Source: CAD feature listing. Evaluate the final solid. Frame: model axes, mm. A direction names the side the tool comes from. Give positions to 0.01 mm unless a question says otherwise; leave off trailing zeros. Order: outer loops, then holes, each group sorted by start corner. A loop starts at its lowest first (then second) coordinate and runs counter-clockwise, first axis right, second up. Notation, with made-up numbers: (78.25, -26) -> (115.25, -26) arc R8 cw to (115.25, -21) -> close; hole circle Ø10 at (-4.5, 45.25). An arc over 180 degrees is marked (long way). Answer in a Markdown table with one row per item.
```python
from build123d import *

# Parameters (mm, degrees)
SKETCH1_R           = 20
BOSS_EXTRUDE1_DEPTH = 2
SKETCH2_R           = 18.25
BOSS_EXTRUDE2_DEPTH = 10
BOSS_EXTRUDE2_TAPER = 3
SKETCH3_R           = 11.5
BOSS_EXTRUDE3_DEPTH = 9.5
FILLET1_R           = 1


with BuildPart() as part:
    # Sketch1 → Boss-Extrude1 (new body)
    with BuildSketch(Plane(origin=(0, 0, 0), x_dir=(1, 0, 0), z_dir=(0, 1, 0))):
        with Locations(Location((0, 0, 0), (0, 0, 270))):
            Circle(SKETCH1_R)
    extrude(amount=BOSS_EXTRUDE1_DEPTH)

    # Sketch2 → Boss-Extrude2 (add)
    with BuildSketch(Plane(origin=(0, 2, 0), x_dir=(1, 0, 0), z_dir=(0, 1, 0))):
        Circle(SKETCH2_R)
    extrude(amount=BOSS_EXTRUDE2_DEPTH, taper=BOSS_EXTRUDE2_TAPER)

    # Sketch3 → Boss-Extrude3 (add)
    with BuildSketch(Plane(origin=(0, 12, 0), x_dir=(1, 0, 0), z_dir=(0, 1, 0))):
        with Locations(Location((0, 0, 0), (0, 0, 270))):
            Circle(SKETCH3_R)
    extrude(amount=BOSS_EXTRUDE3_DEPTH)

    # Fillet1
    fillet1_edges = [part.edges().sort_by_distance(p)[0] for p in [
        (0, 21.5, -11.5),
        (0, 2, -20),
        (-17.725922207, 12, 0),
    ]]
    fillet(fillet1_edges, radius=FILLET1_R)


solid = part.part
```
(1) Access query for faces 1 (the flat face through (0, 21.5, 0)), 2 (the flat face through (17, 2, -7.1)). Directions: +Z, -Z, +X, -X, +Y, -Y. A direction counts if a zero-diameter tool reaches every point of the face in a straight line with its end or side. Return the directions, or none.
A:
| item | result |
|---|---|
| face 1 | +Z, -Z, +X, -X, +Y |
| face 2 | +Y |
(2) Section query B-B (y = 15.25). Return the cut outline in (x, z), plus the area to 3 significant figures.
A:
| item | result |
|---|---|
| outline | circle Ø23 at (0, 0) |
| area | 415 mm^2 |
(3) Ray query, probe 1 along Z at (x, y) = (6.5, 7); probe 2 along Y at (x, z) = (9, 9); probe 3 along Y at (x, z) = (15, -11.5). Return the intervals inside material, ascending.
A:
| item | result |
|---|---|
| probe 1 | z = -16.77 to 16.77 |
| probe 2 | y = 0 to 12 |
| probe 3 | y = 0 to 2 |
(4) Section query C-C (y = 5.25). Return the cut outline in (x, z).
A:
| item | result |
|---|---|
| outline | circle Ø36.16 at (0, 0) |
(5) First-contact query: pin 1 Ø2 at (x, y) = (15, 6) entering from -Z; pin 2 Ø8 at (x, y) = (-1.5, 5.5) entering from +Z; pin 3 Ø1.5 at (y, z) = (18, 9.5) entering from -X. Flat tips, straight axial feed; report the tip coordinate or a pass-through.
A:
| item | result |
|---|---|
| pin 1 | stops at z = -11.38 |
| pin 2 | stops at z = 19.82 |
| pin 3 | stops at x = -7.46 |
(6) Section query A-A (x = 0). Return the cut outline in (y, z).
A:
| item | result |
|---|---|
| outline | (0, -20) -> (1, -20) arc R1 ccw to (2, -19) -> (2, -18.25) -> (11.05, -17.78) arc R1 ccw to (12, -16.78) -> (12, -11.5) -> (20.5, -11.5) arc R1 ccw to (21.5, -10.5) -> (21.5, 10.5) arc R1 ccw to (20.5, 11.5) -> (12, 11.5) -> (12, 16.78) arc R1 ccw to (11.05, 17.78) -> (2, 18.25) -> (2, 19) arc R1 ccw to (1, 20) -> (0, 20) -> close |
